Here's how the part is built. I have some questions about the finished solid (model axes, mm). A direction names the side the tool comes from. Round coordinates to 2 decimals unless told otherwise and drop trailing zeros. Write each loop counter-clockwise with the first axis right and the second up, starting at its lowest first coordinate (ties: lowest second). Pieces come first, ordered by that corner, then holes. Notation, with made-up numbers: (-2, 0.5) -> (52, 0.5) arc R29 cw to (52, 22.5) -> close; hole circle Ø10 at (22, 65.5). An arc over 180 degrees is marked (long way). Answer in a Markdown table with one row per item.
from build123d import *

# Parameters (mm, degrees)
SKETCH1_W                        = 20
SKETCH1_H                        = 20
BOSS_EXTRUDE1_DEPTH              = 30
F_3_0MM_DOWEL_HOLE1_D            = 3
F_3_0MM_DOWEL_HOLE1_DEPTH        = 20
F_3_0MM_DOWEL_HOLE1_CSINK_D      = 3.05
F_3_0MM_DOWEL_HOLE1_CSINK_ANGLE  = 90
F_3_0MM_DOWEL_HOLE1_TIP          = 0.901290929
F_3_0MM_DOWEL_HOLE2_D            = 3
F_3_0MM_DOWEL_HOLE2_DEPTH        = 12
F_3_0MM_DOWEL_HOLE2_CSINK_D      = 3.05
F_3_0MM_DOWEL_HOLE2_CSINK_ANGLE  = 90
F_3_0MM_DOWEL_HOLE2_TIP          = 0.901290929
F_3_0MM_DOWEL_HOLE3_D            = 3
F_3_0MM_DOWEL_HOLE3_DEPTH        = 20
F_3_0MM_DOWEL_HOLE3_CSINK_D      = 3.05
F_3_0MM_DOWEL_HOLE3_CSINK_ANGLE  = 90
F_3_0MM_DOWEL_HOLE3_TIP          = 0.901290929
F_10_0MM_DOWEL_HOLE1_D           = 10
F_10_0MM_DOWEL_HOLE1_DEPTH       = 17
F_10_0MM_DOWEL_HOLE1_CSINK_D     = 10.05
F_10_0MM_DOWEL_HOLE1_CSINK_ANGLE = 90
F_10_0MM_DOWEL_HOLE1_TIP         = 3.004303095


with BuildPart() as part:
    # Sketch1 → Boss-Extrude1 (new body)
    with BuildSketch(Plane(origin=(0, 0, 0), x_dir=(1, 0, 0), z_dir=(0, 1, 0))):
        with Locations((10, -8.099538279)):
            Rectangle(SKETCH1_W, SKETCH1_H)
    extrude(amount=BOSS_EXTRUDE1_DEPTH)

    # Ø3.0mm Dowel Hole1
    with Locations(Plane(origin=(0, 0, -1.900461721), x_dir=(-1, 0, 0), z_dir=(0, 0, -1))):
        with Locations((-16, 20)):
            CounterSinkHole(F_3_0MM_DOWEL_HOLE1_D / 2, F_3_0MM_DOWEL_HOLE1_CSINK_D / 2, depth=F_3_0MM_DOWEL_HOLE1_DEPTH, counter_sink_angle=F_3_0MM_DOWEL_HOLE1_CSINK_ANGLE)
            with Locations((0, 0, -(F_3_0MM_DOWEL_HOLE1_DEPTH + F_3_0MM_DOWEL_HOLE1_TIP / 2))):  # 118° drill point
                Cone(0, F_3_0MM_DOWEL_HOLE1_D / 2, F_3_0MM_DOWEL_HOLE1_TIP, mode=Mode.SUBTRACT)

    # Ø3.0mm Dowel Hole2
    with Locations(Plane.ZY):
        with Locations((8.099538279, 25)):
            CounterSinkHole(F_3_0MM_DOWEL_HOLE2_D / 2, F_3_0MM_DOWEL_HOLE2_CSINK_D / 2, depth=F_3_0MM_DOWEL_HOLE2_DEPTH, counter_sink_angle=F_3_0MM_DOWEL_HOLE2_CSINK_ANGLE)
            with Locations((0, 0, -(F_3_0MM_DOWEL_HOLE2_DEPTH + F_3_0MM_DOWEL_HOLE2_TIP / 2))):  # 118° drill point
                Cone(0, F_3_0MM_DOWEL_HOLE2_D / 2, F_3_0MM_DOWEL_HOLE2_TIP, mode=Mode.SUBTRACT)

    # Ø3.0mm Dowel Hole3
    with Locations(Plane(origin=(0, 30, 0), x_dir=(1, 0, 0), z_dir=(0, 1, 0))):
        with Locations((8, -4.099538279)):
            CounterSinkHole(F_3_0MM_DOWEL_HOLE3_D / 2, F_3_0MM_DOWEL_HOLE3_CSINK_D / 2, depth=F_3_0MM_DOWEL_HOLE3_DEPTH, counter_sink_angle=F_3_0MM_DOWEL_HOLE3_CSINK_ANGLE)
            with Locations((0, 0, -(F_3_0MM_DOWEL_HOLE3_DEPTH + F_3_0MM_DOWEL_HOLE3_TIP / 2))):  # 118° drill point
                Cone(0, F_3_0MM_DOWEL_HOLE3_D / 2, F_3_0MM_DOWEL_HOLE3_TIP, mode=Mode.SUBTRACT)

    # Ø10.0mm Dowel Hole1
    with Locations(Plane(origin=(20, 0, 0), x_dir=(0, 0, -1), z_dir=(1, 0, 0))):
        with Locations((-8.099538279, 8)):
            CounterSinkHole(F_10_0MM_DOWEL_HOLE1_D / 2, F_10_0MM_DOWEL_HOLE1_CSINK_D / 2, depth=F_10_0MM_DOWEL_HOLE1_DEPTH, counter_sink_angle=F_10_0MM_DOWEL_HOLE1_CSINK_ANGLE)
            with Locations((0, 0, -(F_10_0MM_DOWEL_HOLE1_DEPTH + F_10_0MM_DOWEL_HOLE1_TIP / 2))):  # 118° drill point
                Cone(0, F_10_0MM_DOWEL_HOLE1_D / 2, F_10_0MM_DOWEL_HOLE1_TIP, mode=Mode.SUBTRACT)


solid = part.part
1) I want a section at B-B, the plane x = 16. List the corners of the cut face in (y, z) for me (3 decimals), and give its area (3 significant figures).
Response:
| item | result |
|---|---|
| outline | (0, -1.9) -> (18.475, -1.9) -> (18.5, -1.875) -> (18.5, 18.1) -> (0, 18.1) -> close; (21.5, -1.875) -> (21.525, -1.9) -> (30, -1.9) -> (30, 18.1) -> (21.5, 18.1) -> close; hole circle Ø10 at (8, 8.1) |
| area | 461 mm^2 |
2) I need wall thicknesses on line 1 (Z direction, x = 8, y = 25); line 2 (Z direction, x = 15.25, y = 8); line 3 (Y direction, x = 17, z = 4). Which ranges of each line are inside material? Lowest first, please. Write a range as [from, to].
Response:
| item | result |
|---|---|
| line 1 | z = [-1.9, 2.6], [5.6, 6.6], [9.6, 18.1] |
| line 2 | z = [-1.9, 3.1], [13.1, 18.1] |
| line 3 | y = [0, 5.14], [10.86, 18.88], [21.12, 30] |
3) I want a section at D-D, the plane y = 28. List the corners of the cut face in (x, z) for me, and give its area (3 significant figures).
Response:
| item | result |
|---|---|
| outline | (0, -1.9) -> (20, -1.9) -> (20, 18.1) -> (0, 18.1) -> close; hole circle Ø3 at (8, 4.1) |
| area | 393 mm^2 |
4) Which directions (+Z, -Z, +X, -X, +Y, -Y) give clear straight access to the entire face, cutting with the end or side of a thin tool? Please do faces 1 (the face through (0.52, 8.26, 7.27)), 2 (the face through (6.096, 26.487, 8.295)), 3 (the face through (8, 9.7, 3.1)).
Response:
| item | result |
|---|---|
| face 1 | +X |
| face 2 | -X |
| face 3 | +Y |
5) I want a section at A-A, the plane y = 20. List the corners of the cut face in (x, z) for me (3 decimals).
Response:
| item | result |
|---|---|
| outline | (0, -1.9) -> (14.475, -1.9) -> (14.5, -1.875) -> (14.5, 18.1) -> (0, 18.1) -> close; (17.5, -1.875) -> (17.525, -1.9) -> (20, -1.9) -> (20, 18.1) -> (17.5, 18.1) -> close; hole circle Ø3 at (8, 4.1) |
6) For pin 1 (2.5 mm diameter, centred on x = 8, z = 4.1, fed in from +Y); pin 2 (8 mm diameter, centred on y = 8, z = 8.1, fed in from +X), each with a flat end and sliding along its axis, tell me the tip position at first contact or that it passes through.
Response:
| item | result |
|---|---|
| pin 1 | stops at y = 9.85 |
| pin 2 | stops at x = 2.4 |
7) We'd pull the mould along Y, two halves only. Please class faces 4 (the face through (8.195, 19.848, 2.612)), 5 (the face through (11.369, 6.085, 12.718)), 6 (the face through (10, 0, 8)): +Y half, -Y half, draft (parallel to the pull), parting line (faces both ways), or undercut.
Response:
| item | result |
|---|---|
| face 4 | draft |
| face 5 | undercut |
| face 6 | -Y half |
8) I want a section at C-C, the plane x = 18. List the corners of the cut face in (y, z) for me.
Response:
| item | result |
|---|---|
| outline | (0, -1.9) -> (30, -1.9) -> (30, 18.1) -> (0, 18.1) -> close; hole circle Ø10 at (8, 8.1) |
